```python
from build123d import *

# Parameters (mm, degrees)
SKETCH1_R               = 78.359
SKETCH1_R_2             = 76.1746
BOSS_EXTRUDE1_DEPTH     = 12.7
CUT_SWEEP1_START        = -78.35900006
CUT_SWEEP1_OUTLINE_R    = 2.749999961
CUT_SWEEP1_DEPTH        = 2.234055593
MIRROR2_START           = -78.35900006
MIRROR2_COPY_1_SKETCH_R = 2.749999961
MIRROR2_COPY_1_DEPTH    = 2.234055593
SKETCH18_R              = 2.749999961
SKETCH18_W              = 10.000000066
SKETCH18_H              = 6.99999997
CUT_EXTRUDE1_DEPTH      = 112.54172222
SKETCH18_3_R            = 2.749999961
SKETCH18_3_W            = 10.000000066
SKETCH18_3_H            = 6.99999997
CUT_EXTRUDE2_DEPTH      = 112.541722222


# Read off the part's stored shape, not the designer's step: Cut-Sweep1
with BuildPart() as part:
    # Sketch1 → Boss-Extrude1 (new, symmetric)
    with BuildSketch(Plane(origin=(0, 0, 0), x_dir=(1, 0, 0), z_dir=(0, 1, 0))):
        with Locations(Location((0, 0, 0), (0, 0, 270))):
            Circle(SKETCH1_R)
        with Locations(Location((0, 0, 0), (0, 0, 270))):
            Circle(SKETCH1_R_2, mode=Mode.SUBTRACT)
    extrude(amount=BOSS_EXTRUDE1_DEPTH, both=True)

    # Cut-Sweep1 outline → Cut-Sweep1 (cut)
    with BuildSketch(Plane(origin=(0, 0, 0), x_dir=(0.99734525831366, 0, -0.0728178255598082), z_dir=(0.0728178255598082, 0, 0.99734525831366)).offset(CUT_SWEEP1_START)):
        Circle(CUT_SWEEP1_OUTLINE_R)
    cut_sweep1 = extrude(amount=CUT_SWEEP1_DEPTH, mode=Mode.SUBTRACT)

    # Mirror1: Cut-Sweep1 across plane
    add(cut_sweep1.mirror(Plane(origin=(0, 0, 0), x_dir=(0, 0, 1), z_dir=(1, 0, 0))), mode=Mode.SUBTRACT)

    # Mirror2: Cut-Sweep1 across plane
    add(cut_sweep1.mirror(Plane.XY), mode=Mode.SUBTRACT)

    # Mirror2 copy 1 sketch → Mirror2 copy 1 (cut)
    with BuildSketch(Plane(origin=(0, 0, 0), x_dir=(-0.99734525831366, 0, 0.0728178255598082), z_dir=(-0.0728178255598082, 0, -0.99734525831366)).offset(MIRROR2_START)):
        Circle(MIRROR2_COPY_1_SKETCH_R)
    extrude(amount=MIRROR2_COPY_1_DEPTH, mode=Mode.SUBTRACT)

    # Sketch18 → Cut-Extrude1 (cut, through all)
    with BuildSketch(Plane.XY):
        with Locations(Location((0, 3.81, 0), (0, 0, 90))):
            Circle(SKETCH18_R)
        with Locations((0, -8.579999985)):
            Rectangle(SKETCH18_W, SKETCH18_H)
    extrude(amount=-CUT_EXTRUDE1_DEPTH, mode=Mode.SUBTRACT)

    # Sketch18<3> → Cut-Extrude2 (cut, through all)
    with BuildSketch(Plane.XY):
        with Locations(Location((0, -3.81, 0), (0, 0, 269.999999951))):
            Circle(SKETCH18_3_R)
        with Locations((0, 8.579999985)):
            Rectangle(SKETCH18_3_W, SKETCH18_3_H)
    extrude(amount=CUT_EXTRUDE2_DEPTH, mode=Mode.SUBTRACT)


solid = part.part
```
Model file for the job. Use its own axes, mm. A direction names the side the tool comes from. Give positions to 0.01 mm unless a question says otherwise; leave off trailing zeros. Order: outer loops, then holes, each group sorted by start corner. A loop starts at its lowest first (then second) coordinate and runs counter-clockwise, first axis right, second up.
1) Saw through at B-B, the plane x = 45. Write the cut outline in (y, z).
2) Wall check: probe 1 along Y at (x, z) = (0, 77.1); probe 2 along X at (y, z) = (6, 0); probe 3 along Z at (x, y) = (0, 3.25). Give the ranges that are in metal, low to high.
3) Mould opens along X. For faces 1 (the cylindrical face through (-0.83, 6.43, -77.23)), 2 (the flat face through (76, 12.7, -12)), 3 (the cylindrical face through (23.54, 0.18, 74.74)) say: +X half, -X half, draft (parallel to the pull), parting line (faces both ways), or undercut.
4) Pin check, flat tips, straight feed: pin 1 (3.5 mm diameter, centred on x = 0, y = -3.81, fed in from +Z); pin 2 (1.5 mm diameter, centred on x = -59.5, z = 54.5, fed in from -Y); pin 3 (5 mm diameter, centred on x = 0, y = 3.81, fed in from -Z); pin 4 (1.5 mm diameter, centred on y = 1, z = -51, fed in from +X). Stop position of each tip, or through.
5) 3-axis set-ups, long thin cutter, end or side, ignore diameter. For faces 4 (the cylindrical face through (2.727, -3.452, 77.226)), 5 (the cylindrical face through (7.802, -1.673, 76.894)): which of +Z, -Z, +X, -X, +Y, -Y reach the whole face in a straight line?
6) Saw through at A-A, the plane z = 50. Write the cut outline in (x, y).
Computed:
1. outline: (-12.7, -64.15) - (12.7, -64.15) - (12.7, -61.46) - (-12.7, -61.46) - close; (-12.7, 61.46) - (12.7, 61.46) - (12.7, 64.15) - (-12.7, 64.15) - close
2. probe 1: y = -12.7 to -6.56, -1.06 to 5.08, 12.08 to 12.7
2. probe 2: x = -78.36 to -76.17, 76.17 to 78.36
2. probe 3: z = 76.17 to 78.36
3. face 1: undercut
3. face 2: draft
3. face 3: parting line
4. pin 1: stops at z = -76.15
4. pin 2: passes through
4. pin 3: stops at z = 76.13
4. pin 4: stops at x = 60.13
5. face 4: +Z
5. face 5: none
6. outline: (-60.33, -12.7) - (-57.47, -12.7) - (-57.47, 12.7) - (-60.33, 12.7) - close; (57.47, -12.7) - (60.33, -12.7) - (60.33, 12.7) - (57.47, 12.7) - close
